Work out the finished part from the listing and answer in its coordinate system (mm). A direction names the side the tool comes from. Round coordinates to 2 decimals unless told otherwise and drop trailing zeros. Order: outer loops, then holes, each group sorted by start corner. A loop starts at its lowest first (then second) coordinate and runs counter-clockwise, first axis right, second up.
from build123d import *

# Parameters (mm, degrees)
SKETCH_W        = 52
SKETCH_H        = 24
PAD_DEPTH       = 2
SKETCH001_R     = 1.45
POCKET_DEPTH    = 2.001
SKETCH002_R     = 2.85
SKETCH002_R_2   = 1.45
PAD001_DEPTH    = 3
POCKET001_DEPTH = 2.001


with BuildPart() as part:
    # Sketch → Pad (new body)
    with BuildSketch(Plane.XY):
        Rectangle(SKETCH_W, SKETCH_H)
    extrude(amount=PAD_DEPTH)

    # Sketch001 (on Face6 of Pad) → Pocket (cut, through all)
    with BuildSketch(Plane.XY.offset(2)):
        with Locations((-22.9, 8.75)):
            Circle(SKETCH001_R)
        with Locations((22.9, 8.75)):
            Circle(SKETCH001_R)
        with Locations((22.9, -8.75)):
            Circle(SKETCH001_R)
        with Locations((-22.9, -8.75)):
            Circle(SKETCH001_R)
    extrude(amount=-POCKET_DEPTH, mode=Mode.SUBTRACT)

    # Sketch002 (on Face5 of Pocket) → Pad001 (join)
    with BuildSketch(Plane.XY.offset(2)):
        with Locations((-22.9, 8.75)):
            Circle(SKETCH002_R)
        with Locations((-22.9, 8.75)):
            Circle(SKETCH002_R_2, mode=Mode.SUBTRACT)
        with Locations((22.9, 8.75)):
            Circle(SKETCH002_R)
        with Locations((22.9, 8.75)):
            Circle(SKETCH002_R_2, mode=Mode.SUBTRACT)
        with Locations((22.9, -8.75)):
            Circle(SKETCH002_R)
        with Locations((22.9, -8.75)):
            Circle(SKETCH002_R_2, mode=Mode.SUBTRACT)
        with Locations((-22.9, -8.75)):
            Circle(SKETCH002_R)
        with Locations((-22.9, -8.75)):
            Circle(SKETCH002_R_2, mode=Mode.SUBTRACT)
    extrude(amount=PAD001_DEPTH)

    # Sketch003 (on Face5 of Pad001) → Pocket001 (cut, through all)
    with BuildSketch(Plane.XY.offset(2)):
        with BuildLine():
            ThreePointArc((-15.027266, 8), (-23.027266, 0), (-15.027266, -8))
            Line((-15.027266, -8), (15.027266, -8))
            ThreePointArc((15.027266, -8), (23.027266, 0), (15.027266, 8))
            Line((15.027266, 8), (-15.027266, 8))
        make_face()
    extrude(amount=-POCKET001_DEPTH, mode=Mode.SUBTRACT)


solid = part.part
Item 1: Find the intervals of material crossed by line 1 along Y through (x, z) = (-22.9, 3.65); line 2 along Y through (x, z) = (2, 1); line 3 along X through (y, z) = (-7.5, 3.8), in increasing order.
Item 2: Find section A-A (z = 4.2). Write down the section's boundary in (x, y).
Item 3: Given pin 1 (12 mm diameter, centred on x = 14.5, y = -5, fed in from +Z), flat-ended and moving along its own axis, determine where the tip first touches the part or whether it passes through.
Item 4: Find section B-B (x = -14.5). Write down the section's boundary in (y, z), plus the area to 3 significant figures.
Item 5: A tool of negligible diameter and unlimited length cuts with its end or side. For faces 1 (the face through (23.025, -0.176, 1.014)), 2 (the face through (-0.4, 8.2, 2)), 3 (the face through (24.1, 7.5, 5)), from which of +Z, -Z, +X, -X, +Y, -Y can it reach the whole face along a straight path? Write none if from no direction.
Item 6: Find section D-D (y = 0). Write down the section's boundary in (x, z), plus the area to 3 significant figures.
Item 7: Find section C-C (y = -8.75). Write down the section's boundary in (x, z), plus the area to 3 significant figures.
Item 8: For a pull along X with two mould halves and no side action, classify faces 4 (the face through (0, 12, 1)), 5 (the face through (-26, 0, 1)), 6 (the face through (0, -8, 1)) as released by +X, released by -X, zero draft, split by the parting line, or undercut.
Model answer:
1. line 1: y = -11.6 to -10.2, -7.3 to -5.9, 5.9 to 7.3, 10.2 to 11.6
1. line 2: y = -12 to -8, 8 to 12
1. line 3: x = -25.46 to -23.63, -22.17 to -20.34, 20.34 to 22.17, 23.63 to 25.46
2. outline: circle Ø5.7 at (-22.9, -8.75); circle Ø5.7 at (-22.9, 8.75); circle Ø5.7 at (22.9, -8.75); circle Ø5.7 at (22.9, 8.75); hole circle Ø2.9 at (-22.9, -8.75); hole circle Ø2.9 at (-22.9, 8.75); hole circle Ø2.9 at (22.9, -8.75); hole circle Ø2.9 at (22.9, 8.75)
3. pin 1: stops at z = 2
4. outline: (-12, 0) - (-8, 0) - (-8, 2) - (-12, 2) - close; (8, 0) - (12, 0) - (12, 2) - (8, 2) - close
4. area: 16.0 mm2
5. face 1: +Z, -Z
5. face 2: +Z
5. face 3: +Z, +X, -X, +Y, -Y
6. outline: (-26, 0) - (-23.03, 0) - (-23.03, 2) - (-26, 2) - close; (23.03, 0) - (26, 0) - (26, 2) - (23.03, 2) - close
6. area: 11.9 mm2
7. outline: (-26, 0) - (-24.35, 0) - (-24.35, 5) - (-25.75, 5) - (-25.75, 2) - (-26, 2) - close; (-21.45, 0) - (21.45, 0) - (21.45, 5) - (20.05, 5) - (20.05, 2) - (-20.05, 2) - (-20.05, 5) - (-21.45, 5) - close; (24.35, 0) - (26, 0) - (26, 2) - (25.75, 2) - (25.75, 5) - (24.35, 5) - close
7. area: 109 mm2
8. face 4: zero draft
8. face 5: released by -X
8. face 6: undercut
